Study the drawing (mm; zero at the part's minimum x, y, z) and answer. Coordinates: 2 decimals unless noted, no trailing zeros. Loops run counter-clockwise (first coordinate to the right, second up) from the corner with the lowest first, then second, coordinate; pieces in that order, holes last. Notation, with made-up numbers: (40, 14.5) -> (74, 14.5) arc R28 cw to (74, 53.5) -> close; hole circle Ø7 at (6, 11). An arc over 180 degrees is marked (long way). One line per question, with ' | ' between items.
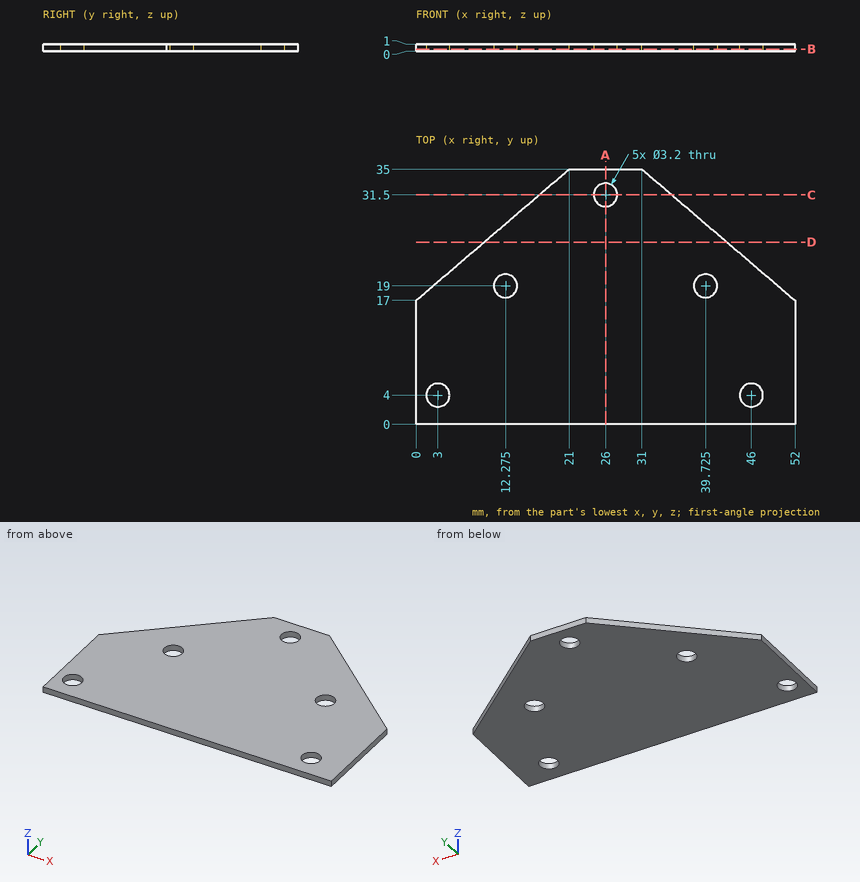
1) Find section B-B (z = 0.3). Write down the section's boundary in (x, y) (3 decimals), plus the area to 3 significant figures.
Check values:
outline: (0, 0) -> (52, 0) -> (52, 17) -> (31, 35) -> (21, 35) -> (0, 17) -> close; hole circle Ø3.2 at (3, 4); hole circle Ø3.2 at (12.275, 19); hole circle Ø3.2 at (26, 31.5); hole circle Ø3.2 at (39.725, 19); hole circle Ø3.2 at (46, 4) | area: 1,400 mm^2
2) Find section A-A (x = 26). Write down the section's boundary in (y, z).
Check values:
outline: (0, 0) -> (29.9, 0) -> (29.9, 1) -> (0, 1) -> close; (33.1, 0) -> (35, 0) -> (35, 1) -> (33.1, 1) -> close
3) A flat-ended cylindrical pin translates along its axis: pin 1 (3 mm diameter, centred on x = 3, y = 4, fed in from +Z). Find the tip coordinate at first contact, or state that the pin passes through.
Check values:
pin 1: passes through
4) Find section D-D (y = 25). Write down the section's boundary in (x, z).
Check values:
outline: (9.33, 0) -> (42.67, 0) -> (42.67, 1) -> (9.33, 1) -> close
5) Find section C-C (y = 31.5). Write down the section's boundary in (x, z).
Check values:
outline: (16.92, 0) -> (24.4, 0) -> (24.4, 1) -> (16.92, 1) -> close; (27.6, 0) -> (35.08, 0) -> (35.08, 1) -> (27.6, 1) -> close
6) Find the intervals of material crossed by line 1 along Y through (x, z) = (26, 0.4); line 2 along X through (y, z) = (3, 0.5); line 3 along Y through (x, z) = (46, 0.4), in increasing order.
Check values:
line 1: y = 0 to 29.9, 33.1 to 35 | line 2: x = 0 to 1.75, 4.25 to 44.75, 47.25 to 52 | line 3: y = 0 to 2.4, 5.6 to 22.14
